Verification items for the finished model (mm, model axes). Face numbers are marked on the shaded views. Coordinates: 2 decimals unless noted, no trailing zeros. Loops run counter-clockwise (first coordinate to the right, second up) from the corner with the lowest first, then second, coordinate; pieces in that order, holes last. Notation, with made-up numbers: (-19.5, 16) -> (2.5, 16) arc R9 ccw to (2.5, 26) -> close; hole circle Ø7 at (13.5, 76.25). An arc over 180 degrees is marked (long way). Answer as a JSON object with one key per item and string values. Group by question number.
Q1. Gauge pin test, flat ends, axial feed: pin 1 Ø3 at (y, z) = (-94, 17.5) entering from +X; pin 2 Ø8 at (x, z) = (107.5, 64) entering from -Y; pin 3 Ø4 at (y, z) = (2, 58) entering from +X. Record the tip position at first contact, or that the pin passes through.
Q2. Release check for a two-part mould opening along Y. For the marked faces 1, 2 and 3 record: released by +Y, released by -Y, zero draft, split by the parting line, or undercut.
Q3. Scan lines: L1, parallel to Y at x = 0, z = 71; L2, parallel to X at y = -98.5, z = 58.5; L3, parallel to Y at x = 49.5, z = 41. Record each from-to range of solid material in increasing order.
Q4. Cross-section at A-A on z = 55.5. Record the boundary of the cut face in (x, y), and give its area (3 significant figures).
```python
from build123d import *

# Parameters (mm, degrees)
F0_R     = 140
F0_R_2   = 120
F1_DEPTH = 3
F2_R     = 123
F2_R_2   = 120
F3_DEPTH = 100
F4_R     = 6
F6_DEPTH = 3.0010001


with BuildPart() as f1:
    # F0 (on Top) → F1 (new body)
    with BuildSketch(Plane.XY):
        Circle(F0_R)
        Circle(F0_R_2, mode=Mode.SUBTRACT)
    extrude(amount=F1_DEPTH)

    # F2 (on face) → F3 (join)
    with BuildSketch(Plane.XY.offset(3)):
        Circle(F2_R)
        Circle(F2_R_2, mode=Mode.SUBTRACT)
    extrude(amount=F3_DEPTH)

    # F4
    f4_edges = [f1.edges().sort_by_distance(p)[0] for p in [
        (-120, 0, 0),
    ]]
    fillet(f4_edges, radius=F4_R)

    # F5 (on face) → F6 (cut, through all)
    with BuildSketch(Plane.XY.offset(3)):
        with BuildLine():
            ThreePointArc((-101.0935386677, -96.8508979806), (-98.9949493661, -98.9949493661), (-96.8508979806, -101.0935386677))
            Line((-96.8508979806, -101.0935386677), (-91.9238815543, -96.1665222414))
            ThreePointArc((-91.9238815543, -96.1665222414), (-91.9238815543, -91.9238815543), (-96.1665222414, -91.9238815543))
            Line((-96.1665222414, -91.9238815543), (-101.0935386677, -96.8508979806))
        make_face()
        with BuildLine():
            ThreePointArc((0, -140), (1.5000861142, -139.9919631324), (3, -139.9678534521))
            Line((3, -139.9678534521), (3, -133))
            ThreePointArc((3, -133), (0, -130), (-3, -133))
            Line((-3, -133), (-3, -139.9678534521))
            ThreePointArc((-3, -139.9678534521), (-1.5000861142, -139.9919631324), (0, -140))
        make_face()
        with BuildLine():
            Line((-133, 3), (-139.9678534521, 3))
            ThreePointArc((-139.9678534521, 3), (-140, 0), (-139.9678534521, -3))
            Line((-139.9678534521, -3), (-133, -3))
            ThreePointArc((-133, -3), (-130, 0), (-133, 3))
        make_face()
        with BuildLine():
            Line((-91.9238815543, 96.1665222414), (-96.8508979806, 101.0935386677))
            ThreePointArc((-96.8508979806, 101.0935386677), (-98.9949493661, 98.9949493661), (-101.0935386677, 96.8508979806))
            Line((-101.0935386677, 96.8508979806), (-96.1665222414, 91.9238815543))
            ThreePointArc((-96.1665222414, 91.9238815543), (-91.9238815543, 91.9238815543), (-91.9238815543, 96.1665222414))
        make_face()
        with BuildLine():
            Line((3, 133), (3, 139.9678534521))
            ThreePointArc((3, 139.9678534521), (0, 140), (-3, 139.9678534521))
            Line((-3, 139.9678534521), (-3, 133))
            ThreePointArc((-3, 133), (0, 130), (3, 133))
        make_face()
        with BuildLine():
            ThreePointArc((96.8508979806, -101.0935386677), (98.9949493661, -98.9949493661), (101.0935386677, -96.8508979806))
            Line((101.0935386677, -96.8508979806), (96.1665222414, -91.9238815543))
            ThreePointArc((96.1665222414, -91.9238815543), (91.9238815543, -91.9238815543), (91.9238815543, -96.1665222414))
            Line((91.9238815543, -96.1665222414), (96.8508979806, -101.0935386677))
        make_face()
        with BuildLine():
            ThreePointArc((139.9678534521, -3), (139.9919631324, -1.5000861142), (140, 0))
            ThreePointArc((140, 0), (139.9919631324, 1.5000861142), (139.9678534521, 3))
            Line((139.9678534521, 3), (133, 3))
            ThreePointArc((133, 3), (130, 0), (133, -3))
            Line((133, -3), (139.9678534521, -3))
        make_face()
        with BuildLine():
            Line((96.1665222414, 91.9238815543), (101.0935386677, 96.8508979806))
            ThreePointArc((101.0935386677, 96.8508979806), (98.9949493661, 98.9949493661), (96.8508979806, 101.0935386677))
            Line((96.8508979806, 101.0935386677), (91.9238815543, 96.1665222414))
            ThreePointArc((91.9238815543, 96.1665222414), (91.9238815543, 91.9238815543), (96.1665222414, 91.9238815543))
        make_face()
    extrude(amount=-F6_DEPTH, mode=Mode.SUBTRACT)


solid = f1.part
```
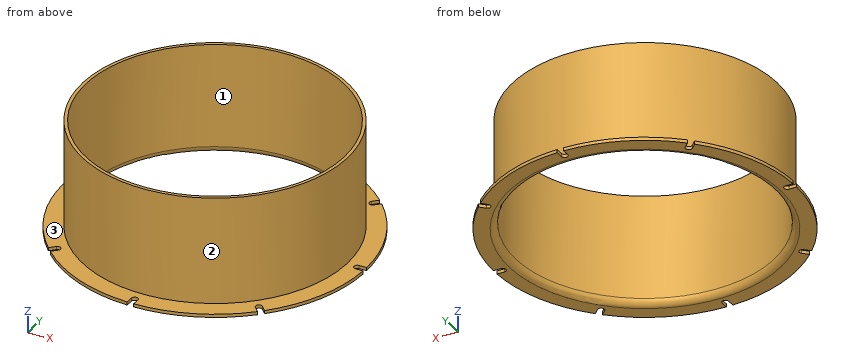
Computed values:
{
 "1": {"pin 1": "stops at x = 81.07", "pin 2": "stops at y = -66.46", "pin 3": "stops at x = 123"},
 "2": {"face 1": "undercut", "face 2": "split by the parting line", "face 3": "zero draft"},
 "3": {"L1": "y = -123 to -120, 120 to 123", "L2": "x = -73.67 to -68.54, 68.54 to 73.67", "L3": "y = -112.6 to -109.31, 109.31 to 112.6"},
 "4": {"outline": "circle Ø246 at (0, 0); hole circle Ø240 at (0, 0)", "area": "2,290 mm²"}
}
